from build123d import *

# Parameters (mm, degrees)
SKETCH_1_W          = 35
SKETCH_1_H          = 10
SKETCH_1_W_2        = 33
SKETCH_1_H_2        = 8
EXTRUDE_1_DEPTH     = 15
SKETCH_2_R          = 1.5
CUT_EXTRUDE_1_DEPTH = 50
SKETCH_3_R          = 4
SKETCH_3_R_2        = 1.5
CUT_EXTRUDE_2_DEPTH = 10


with BuildPart() as part:
    # 草图1 → 凸台-拉伸1 (new, symmetric)
    with BuildSketch(Plane.XY):
        Rectangle(SKETCH_1_W, SKETCH_1_H)
        Rectangle(SKETCH_1_W_2, SKETCH_1_H_2, mode=Mode.SUBTRACT)
    extrude(amount=EXTRUDE_1_DEPTH, both=True)

    # 草图2 → 切除-拉伸1 (cut)
    with BuildSketch(Plane(origin=(17.5, 0, 0), x_dir=(0, 0, -1), z_dir=(1, 0, 0))):
        with Locations((11.5, 0)):
            Circle(SKETCH_2_R)
        with Locations((-11.5, 0)):
            Circle(SKETCH_2_R)
    extrude(amount=-CUT_EXTRUDE_1_DEPTH, mode=Mode.SUBTRACT)

    # 草图3 → 切除-拉伸2 (cut)
    with BuildSketch(Plane(origin=(0, 5, 0), x_dir=(1, 0, 0), z_dir=(0, 1, 0))):
        with Locations(Location((0, 0, 0), (0, 0, 270))):
            Circle(SKETCH_3_R)
        with Locations(Location((-4.5, 7.794228634, 0), (0, 0, 270))):
            Circle(SKETCH_3_R_2)
        with Locations(Location((4.5, 7.794228634, 0), (0, 0, 270))):
            Circle(SKETCH_3_R_2)
        with Locations(Location((9, 0, 0), (0, 0, 270))):
            Circle(SKETCH_3_R_2)
        with Locations(Location((4.5, -7.794228634, 0), (0, 0, 270))):
            Circle(SKETCH_3_R_2)
        with Locations(Location((-4.5, -7.794228634, 0), (0, 0, 270))):
            Circle(SKETCH_3_R_2)
        with Locations(Location((-9, 0, 0), (0, 0, 270))):
            Circle(SKETCH_3_R_2)
    extrude(amount=-CUT_EXTRUDE_2_DEPTH, mode=Mode.SUBTRACT)


solid = part.part
Geometry: final body of the model. Coordinates: model frame, mm. A direction names the side the tool comes from. Give positions to 0.01 mm unless a question says otherwise; leave off trailing zeros. Order: outer loops, then holes, each group sorted by start corner. A loop starts at its lowest first (then second) coordinate and runs counter-clockwise, first axis right, second up. Notation, with made-up numbers: (-8.5, 51) - (14.5, 51) arc R11 ccw to (14.5, 71) - close; hole circle Ø9 at (31.5, 20). An arc over 180 degrees is marked (long way). Use CSV: the item, a comma, the result in double quotes.
1. Mould query, pull axis Y, two halves, no side actions, for faces 1 (the face through (-3.013, -4.493, 7.599)), 2 (the face through (4, -5, -3)), 3 (the face through (-16.5, 0, 0)). Classes: +Y half, -Y half, draft (parallel to the pull), parting line (faces both ways), or undercut.
Answers below:
face 1,"draft"
face 2,"-Y half"
face 3,"undercut"
2. Access query for faces 4 (the face through (3, -4, -3)), 5 (the face through (3.93, 4.51, 9.18)). Directions: +Z, -Z, +X, -X, +Y, -Y. A direction counts if a zero-diameter tool reaches every point of the face in a straight line with its end or side. Return the directions, or none.
Answers below:
face 4,"+Z, -Z"
face 5,"+Y, -Y"
3. Material intervals for line 1 along X through (y, z) = (-4.4, 0); line 2 along Y through (x, z) = (-13, -1); line 3 along Y through (x, z) = (16.85, 11.5), sorted ascending. Write a range as from..to.
Answers below:
line 1,"-17.5..-10.5, -7.5..-4, 4..7.5, 10.5..17.5"
line 2,"-5..-4, 4..5"
line 3,"-5..-1.5, 1.5..5"
4. Section query B-B (z = -11.5). Output: boundary loops of the cut face in (x, y), plus the area to 3 significant figures.
Answers below:
outline,"(-17.5, -5) - (17.5, -5) - (17.5, -1.5) - (16.5, -1.5) - (16.5, -4) - (-16.5, -4) - (-16.5, -1.5) - (-17.5, -1.5) - close; (-17.5, 1.5) - (-16.5, 1.5) - (-16.5, 4) - (16.5, 4) - (16.5, 1.5) - (17.5, 1.5) - (17.5, 5) - (-17.5, 5) - close"
area,"80.0 mm2"
5. Section query C-C (y = -2). Output: boundary loops of the cut face in (x, z).
Answers below:
outline,"(-17.5, -15) - (-16.5, -15) - (-16.5, 15) - (-17.5, 15) - close; (16.5, -15) - (17.5, -15) - (17.5, 15) - (16.5, 15) - close"
6. Section query A-A (x = -4.5). Output: boundary loops of the cut face in (y, z), plus the area to 3 significant figures.
Answers below:
outline,"(-5, -15) - (-4, -15) - (-4, -9.29) - (-5, -9.29) - close; (-5, -6.29) - (-4, -6.29) - (-4, 6.29) - (-5, 6.29) - close; (-5, 9.29) - (-4, 9.29) - (-4, 15) - (-5, 15) - close; (4, -15) - (5, -15) - (5, -9.29) - (4, -9.29) - close; (4, -6.29) - (5, -6.29) - (5, 6.29) - (4, 6.29) - close; (4, 9.29) - (5, 9.29) - (5, 15) - (4, 15) - close"
area,"48.0 mm2"
7. Section query D-D (y = 0). Output: boundary loops of the cut face in (x, z).
Answers below:
outline,"(-17.5, -15) - (-16.5, -15) - (-16.5, -13) - (-17.5, -13) - close; (-17.5, -10) - (-16.5, -10) - (-16.5, 10) - (-17.5, 10) - close; (-17.5, 13) - (-16.5, 13) - (-16.5, 15) - (-17.5, 15) - close; (16.5, -15) - (17.5, -15) - (17.5, -13) - (16.5, -13) - close; (16.5, -10) - (17.5, -10) - (17.5, 10) - (16.5, 10) - close; (16.5, 13) - (17.5, 13) - (17.5, 15) - (16.5, 15) - close"
